Verification items for the finished model (mm, model axes). A direction names the side the tool comes from. Round coordinates to 2 decimals unless told otherwise and drop trailing zeros. Order: outer loops, then holes, each group sorted by start corner. A loop starts at its lowest first (then second) coordinate and runs counter-clockwise, first axis right, second up. Notation, with made-up numbers: (82, 27.25) -> (99, 27.25) arc R16 cw to (99, 35.25) -> close; hole circle Ø2 at (-40, 27). An arc over 180 degrees is marked (long way). Return JSON: item names as keys, results as strings. Group by question number.
Item 1: Sectioned sample at B-B on y = 1. Record the cut outline in (x, z) (1 decimal).
Item 2: Scan lines: probe 1 along Z at (x, y) = (0, 4.75); probe 2 along Z at (x, y) = (-0.6, -5); probe 3 along Y at (x, z) = (-1.15, -2.75). Record each from-to range of solid material in increasing order. Write a range as from..to.
Item 3: Access from +Z, -Z, +X, -X, +Y, -Y to the whole of each face (thin tool, end or side, straight path). Record for faces 1 (the cylindrical face through (-0.34, 0.19, -9.22)), 2 (the flat face through (0, 8, 0)), 3 (the cylindrical face through (-0.207, -9.074, -12.744)).
Item 4: Depth check by flat-ended pin: pin 1 Ø1 at (x, y) = (0.5, -3.5) entering from -Z. Enter the tip coordinate at first touch or a pass-through.
Item 5: Sectioned sample at A-A on z = -3. Record the cut outline in (x, y) (1 decimal).
Autodesk Inventor part; units mm, degrees
ref_plane "YZ Plane" through (0, 0, 0) normal (1, 0, 0) x (0, 1, 0)
ref_plane "XZ Plane" through (0, 0, 0) normal (0, 1, 0) x (-1, 0, 0)
ref_plane "XY Plane" through (0, 0, 0) normal (0, 0, 1) x (1, 0, 0)
sketch "Sketch3" plane through (0, 0, 0) normal (0, 0, 1) x (1, 0, 0)
  circle A0 centre (0, 7.5) radius 1.5875
  point P0 (0, 0)
  dimension "d10" = 3.175
  dimension "d11" = 7.5
sketch "Sketch4" plane through (0, 0, 0) normal (1, 0, 0) x (0, 1, 0)
  line L0 (7.7682, 0) -> (7.7682, -6.35)
  line L1 (7.7682, 0) -> (14.1182, 0) construction
  line L2 (6.1807, -7.9375) -> (-5.6443, -7.9375)
  line L3 (-7.2318, -9.525) -> (-7.2318, -15.875)
  arc A0 (6.1807, -7.9375) -> (7.7682, -6.35) centre (6.1807, -6.35) ccw
  arc A1 (-5.6443, -7.9375) -> (-7.2318, -9.525) centre (-5.6443, -9.525) ccw
  point P0 (0, 0)
  point P1 (7.7682, -7.9375)
  point P2 (-7.2318, -7.9375)
  dimension "d12" = 7.9375
  dimension "d13" = 90
  dimension "d14" = 15
  dimension "d15" = 90
  dimension "d16" = 7.9375
  dimension "d17" = 1.5875
sweep "Sweep2" add profiles "Sketch3" path "Sketch4"
properties part number "crank bar" material "ABS Plastic"
Recorded:
{
 "1": {"outline": "circle Ø3.2 at (0, -7.7)"},
 "2": {"probe 1": "-9.26..-6.08", "probe 2": "-9.14..-6.2", "probe 3": "6.41..8.59"},
 "3": {"face 1": "none", "face 2": "+Z, +X, -X, +Y, -Y", "face 3": "-Z"},
 "4": {"pin 1": "z = -9.26"},
 "5": {"outline": "circle Ø3.2 at (0, 7.5)"}
}
